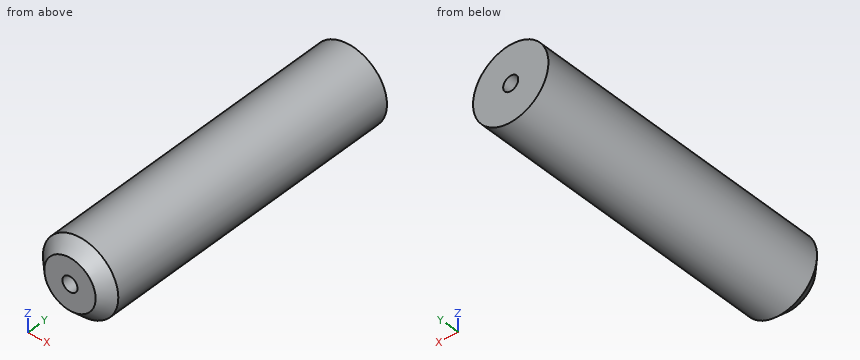
from build123d import *

# Parameters (mm, degrees)
SKETCH1_R           = 12.5
BOSS_EXTRUDE1_DEPTH = 105
SKETCH2_R           = 2.5
CUT_EXTRUDE1_DEPTH  = 105
CHAMFER1_SIZE       = 4


with BuildPart() as part:
    # Sketch1 → Boss-Extrude1 (new body)
    with BuildSketch(Plane(origin=(0, 0, 0), x_dir=(1, 0, 0), z_dir=(0, 1, 0))):
        Circle(SKETCH1_R)
    extrude(amount=BOSS_EXTRUDE1_DEPTH)

    # Sketch2 → Cut-Extrude1 (cut)
    with BuildSketch(Plane(origin=(0, 105, 0), x_dir=(1, 0, 0), z_dir=(0, 1, 0))):
        Circle(SKETCH2_R)
    extrude(amount=-CUT_EXTRUDE1_DEPTH, mode=Mode.SUBTRACT)

    # Chamfer1
    chamfer1_edges = [part.edges().sort_by_distance(p)[0] for p in [
        (-12.5, 0, 0),
    ]]
    chamfer(chamfer1_edges, length=CHAMFER1_SIZE)


solid = part.part
Geometry: final body of the model. Coordinates: model frame, mm. Give positions to 0.01 mm unless a question says otherwise; leave off trailing zeros. Write each loop counter-clockwise with the first axis right and the second up, starting at its lowest first coordinate (ties: lowest second). Pieces come first, ordered by that corner, then holes. Notation, with made-up numbers: (37.5, 37) - (94.5, 37) arc R29 ccw to (94.5, 70) - close; hole circle Ø9 at (71, 26.5). An arc over 180 degrees is marked (long way). Return JSON: item names as keys, results as strings. Group by question number.
1) Section A-A on z = 0. Return the cut outline in (x, y).
2) Line query: line 1 (X direction, y = 67, z = 0); line 2 (X direction, y = 20, z = 1). Output: solid intervals per line, ascending.
3) Section B-B on x = 0. Return the cut outline in (y, z).
4) Section C-C on y = 8.5. Return the cut outline in (x, z).
5) First-contact query: P1, Ø1, axis at x = -5.5, y = 59.5, coming from the +Z side; P2, Ø8, axis at x = 7.5, y = 68, coming from the +Z side; P3, Ø3, axis at y = 54.5, z = -9, coming from the -X side; P4, Ø3, axis at x = 0, z = 0, coming from the +Y side. Flat tips, straight axial feed; report the tip coordinate or a pass-through.
Filled in:
{
 "1": {"outline": "(-12.5, 4) - (-8.5, 0) - (-2.5, 0) - (-2.5, 105) - (-12.5, 105) - close; (2.5, 0) - (8.5, 0) - (12.5, 4) - (12.5, 105) - (2.5, 105) - close"},
 "2": {"line 1": "x = -12.5 to -2.5, 2.5 to 12.5", "line 2": "x = -12.46 to -2.29, 2.29 to 12.46"},
 "3": {"outline": "(0, -8.5) - (4, -12.5) - (105, -12.5) - (105, -2.5) - (0, -2.5) - close; (0, 2.5) - (105, 2.5) - (105, 12.5) - (4, 12.5) - (0, 8.5) - close"},
 "4": {"outline": "circle Ø25 at (0, 0); hole circle Ø5 at (0, 0)"},
 "5": {"P1": "stops at z = 11.46", "P2": "stops at z = 12", "P3": "stops at x = -10", "P4": "passes through"}
}
